from build123d import *

# Parameters (mm, degrees)
SKETCH_1_W             = 5.6
SKETCH_1_H             = 12
EXTRUDE_1_DEPTH        = 175
SKETCH_2_R             = 1.5
CUT_EXTRUDE_1_DEPTH    = 350
SKETCH_3_R             = 5
CUT_EXTRUDE_2_DEPTH    = 350
HOLE_WIZARD_M3_1_D     = 2.5
PATTERN_LINEAR_2_COUNT = 3
PATTERN_LINEAR_2_PITCH = 160


with BuildPart() as part:
    # 草图1 → 凸台-拉伸1 (new, symmetric)
    with BuildSketch(Plane(origin=(0, 0, 0), x_dir=(0, 0, -1), z_dir=(1, 0, 0))):
        with Locations((2.8, 0)):
            Rectangle(SKETCH_1_W, SKETCH_1_H)
    extrude(amount=EXTRUDE_1_DEPTH, both=True)

    # 草图2 → 切除-拉伸1 (cut)
    with BuildSketch(Plane(origin=(175, 0, 0), x_dir=(0, 0, -1), z_dir=(1, 0, 0))):
        with Locations((2.8, 6)):
            Circle(SKETCH_2_R)
        with Locations((2.8, -6)):
            Circle(SKETCH_2_R)
    extrude(amount=-CUT_EXTRUDE_1_DEPTH, mode=Mode.SUBTRACT)

    # 草图3 → 切除-拉伸2 (cut)
    with BuildSketch(Plane(origin=(175, 0, 0), x_dir=(0, 0, -1), z_dir=(1, 0, 0))):
        with Locations((-3, 0)):
            Circle(SKETCH_3_R)
    extrude(amount=-CUT_EXTRUDE_2_DEPTH, mode=Mode.SUBTRACT)

    # M3 螺纹孔1 (through all)
    with Locations(Plane(origin=(0, 0, -5.6), x_dir=(-1, 0, 0), z_dir=(0, 0, -1))):
        with Locations((-160, 0)):
            hole_wizard_m3_1 = Hole(HOLE_WIZARD_M3_1_D / 2)

    # 阵列(线性)2: M3 螺纹孔1 ×3
    with Locations(*[(-i * PATTERN_LINEAR_2_PITCH, 0, 0) for i in range(1, PATTERN_LINEAR_2_COUNT)]):
        add(hole_wizard_m3_1, mode=Mode.SUBTRACT)


solid = part.part
Can you work these out from the model? Positions are in its coordinate system, mm. Round coordinates to 2 decimals unless told otherwise and drop trailing zeros. Order: outer loops, then holes, each group sorted by start corner. A loop starts at its lowest first (then second) coordinate and runs counter-clockwise, first axis right, second up. Notation, with made-up numbers: (7.5, 76.5) - (31.5, 76.5) arc R5 cw to (31.5, 81.5) - close; hole circle Ø3 at (-19, 42). An arc over 180 degrees is marked (long way). Answer in a Markdown table with one row per item.
(1) For P1, Ø2, axis at x = 0, y = 0, coming from the -Z side; P2, Ø2, axis at x = 71.5, y = 1, coming from the +Z side; P3, Ø1.5, axis at x = 124.5, y = -1.5, coming from the +Z side, each with a flat end and sliding along its axis, tell me the tip position at first contact or that it passes through.
From the geometry:
| item | result |
|---|---|
| P1 | passes through |
| P2 | stops at z = -1.58 |
| P3 | stops at z = -1.47 |
(2) Suppose I cut it at A-A, the plane x = 98.5. Please give me the cut outline in (y, z), plus the area to 3 significant figures.
From the geometry:
| item | result |
|---|---|
| outline | (-6, -5.6) - (6, -5.6) - (6, -4.3) arc R1.5 cw to (6, -1.3) - (6, 0) - (4, 0) arc R5 cw to (-4, 0) - (-6, 0) - (-6, -1.3) arc R1.5 cw to (-6, -4.3) - close |
| area | 48.9 mm2 |
(3) If we mould it in two halves opening along Y, with no side actions, what happens to faces 1 (the face through (-175, 0, -3)), 2 (the face through (2, 0, -2))? For each: released by +Y, released by -Y, zero draft, split by the parting line, or undercut.
From the geometry:
| item | result |
|---|---|
| face 1 | zero draft |
| face 2 | undercut |
(4) Please list where these lines run through material, in increasing order: L1, parallel to X at y = 0, z = -2.9; L2, parallel to Y at x = 160, z = -4.45; L3, parallel to Y at x = 0, z = -2.85. Write a range as from..to.
From the geometry:
| item | result |
|---|---|
| L1 | x = -175..-161.25, -158.75..-1.25, 1.25..158.75, 161.25..175 |
| L2 | y = -6..-1.25, 1.25..6 |
| L3 | y = -4.5..-1.25, 1.25..4.5 |
(5) Suppose I cut it at B-B, the plane z = -3.35. Please give me the cut outline in (x, y).
From the geometry:
| item | result |
|---|---|
| outline | (-175, -4.6) - (175, -4.6) - (175, 4.6) - (-175, 4.6) - close; hole circle Ø2.5 at (-160, 0); hole circle Ø2.5 at (0, 0); hole circle Ø2.5 at (160, 0) |
